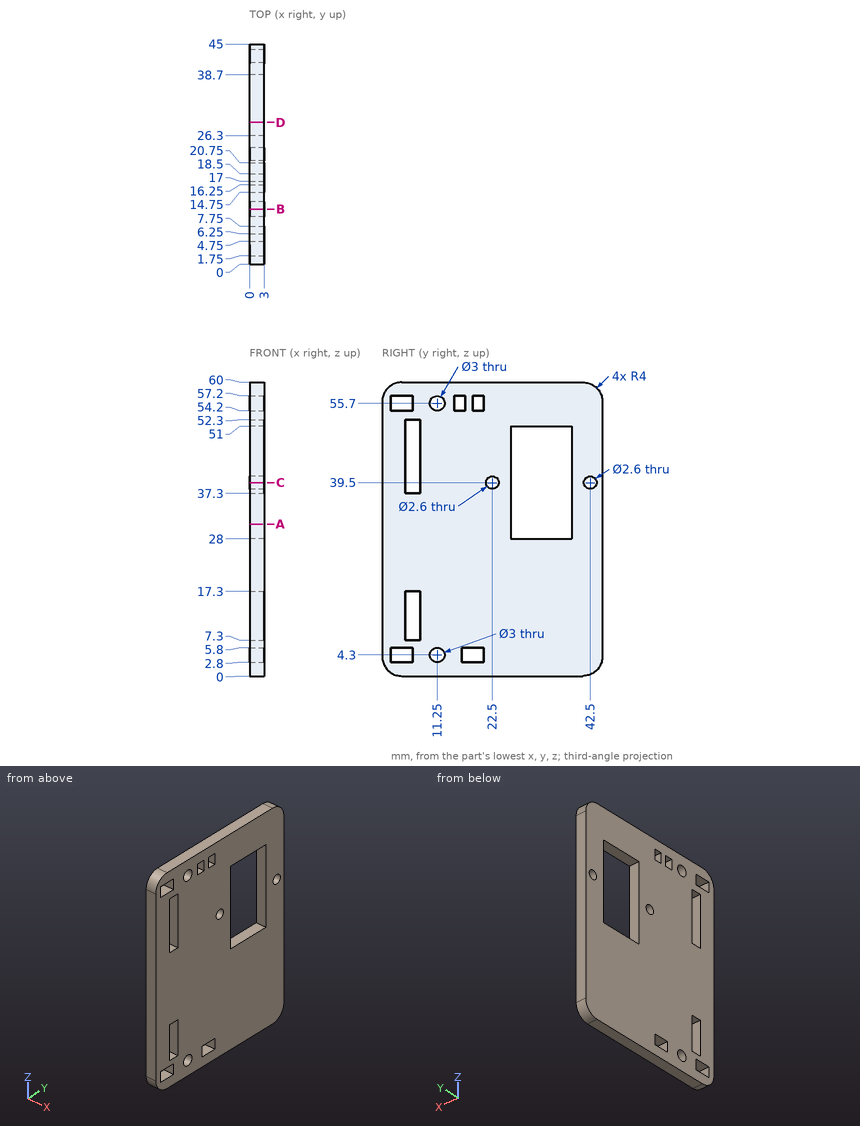
The drawing under review shows one solid part. Ordinate dimensions are in mm from its lowest x, y, z. Give positions to 0.01 mm unless a question says otherwise; leave off trailing zeros. Order: outer loops, then holes, each group sorted by start corner. A loop starts at its lowest first (then second) coordinate and runs counter-clockwise, first axis right, second up. Notation, with made-up numbers: (69.5, 21.25) - (124.5, 21.25) arc R8 ccw to (124.5, 28.25) - close; hole circle Ø9 at (76, 79). An arc over 180 degrees is marked (long way). Answer as a JSON object with one key per item and string values. Group by question number.
Item 1: Clearance check with a flat-ended pin moving along its axis: pin 1 Ø0.9 at (x, y) = (2, 3) entering from +Z. State where the tip first meets the part, or that it passes through.
Item 2: Take a section at C-C on z = 39.5. Give the boundary of the cut face in (x, y).
Item 3: Wall thickness on line 1 along Z through (x, y) = (2.25, 20.5); line 2 along Y through (x, z) = (0.9, 55.7); line 3 along Y through (x, z) = (0.65, 4.3): over which ranges is each line inside the solid? List them lowest first.
Item 4: Take a section at D-D on y = 29. Give the boundary of the cut face in (x, z).
Item 5: Take a section at A-A on z = 31. Give the boundary of the cut face in (x, y), and give its area (3 significant figures).
Item 6: Take a section at B-B on y = 11.25. Give the boundary of the cut face in (x, z).
Reported:
{
 "1": {"pin 1": "z = 59.96"},
 "2": {"outline": "(0, 0) - (3, 0) - (3, 4.75) - (0, 4.75) - close; (0, 7.75) - (3, 7.75) - (3, 21.2) - (0, 21.2) - close; (0, 23.8) - (3, 23.8) - (3, 26.3) - (0, 26.3) - close; (0, 38.7) - (3, 38.7) - (3, 41.2) - (0, 41.2) - close; (0, 43.8) - (3, 43.8) - (3, 45) - (0, 45) - close"},
 "3": {"line 1": "0 to 2.8, 5.8 to 54.2, 57.2 to 60", "line 2": "0 to 1.75, 6.25 to 9.75, 12.75 to 14.75, 17 to 18.5, 20.75 to 45", "line 3": "0 to 1.75, 6.25 to 9.75, 12.75 to 16.25, 20.75 to 45"},
 "4": {"outline": "(0, 0) - (3, 0) - (3, 28) - (0, 28) - close; (0, 51) - (3, 51) - (3, 60) - (0, 60) - close"},
 "5": {"outline": "(0, 0) - (3, 0) - (3, 26.3) - (0, 26.3) - close; (0, 38.7) - (3, 38.7) - (3, 45) - (0, 45) - close", "area": "97.8 mm^2"},
 "6": {"outline": "(0, 0) - (3, 0) - (3, 2.8) - (0, 2.8) - close; (0, 5.8) - (3, 5.8) - (3, 54.2) - (0, 54.2) - close; (0, 57.2) - (3, 57.2) - (3, 60) - (0, 60) - close"}
}
